Design review of the part built by this model. Coordinates are the model's own, in mm. A direction names the side the tool comes from. Round coordinates to 2 decimals unless told otherwise and drop trailing zeros. Loops run counter-clockwise (first coordinate to the right, second up) from the corner with the lowest first, then second, coordinate; pieces in that order, holes last. Notation, with made-up numbers: M 83.5,74 L 90.5,74 A25 ccw 90.5,95 Z; hole C -9.5,-4 d2. An arc over 180 degrees is marked long. One line per item, written item: value. Start each with the question number.
Item 1: We need section B-B (z = 26.5). Write out the cut boundary in (x, y), then the cut area to 3 significant figures.
Item 2: We need section A-A (x = -42.5). Write out the cut boundary in (y, z).
Item 3: Clearance check with flat-ended pins moving along their axes: pin 1 (12 mm diameter, centred on x = 9.5, z = 99.5, fed in from -Y); pin 2 (6 mm diameter, centred on y = -5.5, z = -70.5, fed in from +X); pin 3 (3 mm diameter, centred on x = 64.5, y = -5, fed in from +Z). State where each tip first meets the part, or that it passes through.
Item 4: For line 1 along Z through (x, y) = (101, -2.75); line 2 along Y through (x, z) = (-25, -11), list the stretches that pass through material, from the lowest coordinate up.
Item 5: For faces 1 (the flat face through (15, -8, 62)), 2 (the flat face through (-62, -8, -15)), 3 (the flat face through (-15, -8, 62)), 4 (the flat face through (63, -8, -15)), list the 3-axis set-ups (+Z, -Z, +X, -X, +Y, -Y) from which the entire face can be reached by the end or side of a thin tool; tool diameter is ignored.
from build123d import *

# Parameters (mm, degrees)
F0_W      = 30
F0_H      = 30
F1_DEPTH  = 20
F5_W      = 20
F5_H      = 30
F6_DEPTH  = 110
F4_W      = 30
F4_H      = 20
F7_DEPTH  = 110
F3_W      = 20
F3_H      = 30
F8_DEPTH  = 110
F2_W      = 30
F2_H      = 20
F9_DEPTH  = 110
F10_SIZE2 = 10
F10_SIZE  = 110
F11_R     = 14.99999


# Not quite as in the source:
# - a fillet or chamfer is up to 0.001 mm smaller than in the source, because OpenCascade refuses the exact size


with BuildPart() as f1:
    # F0 (on Front) → F1 (new body)
    with BuildSketch(Plane.XZ):
        Rectangle(F0_W, F0_H)
    extrude(amount=F1_DEPTH)

    # F5 (on face) → F6 (join)
    with BuildSketch(Plane.YZ.offset(15)):
        with Locations((-10, 0)):
            Rectangle(F5_W, F5_H)
    extrude(amount=F6_DEPTH)

    # F4 (on face) → F7 (join)
    with BuildSketch(Plane.XY.offset(15)):
        with Locations((0, -10)):
            Rectangle(F4_W, F4_H)
    extrude(amount=F7_DEPTH)

    # F3 (on face) → F8 (join)
    with BuildSketch(Plane(origin=(-15, 0, 0), x_dir=(0, -1, 0), z_dir=(-1, 0, 0))):
        with Locations((10, 0)):
            Rectangle(F3_W, F3_H)
    extrude(amount=F8_DEPTH)

    # F2 (on face) → F9 (join)
    with BuildSketch(Plane(origin=(0, 0, -15), x_dir=(1, 0, 0), z_dir=(0, 0, -1))):
        with Locations((0, 10)):
            Rectangle(F2_W, F2_H)
    extrude(amount=F9_DEPTH)

    # F10
    f10_edges = [f1.edges().sort_by_distance(p)[0] for p in [
        (-125, -20, 0),
        (0, -20, -125),
        (125, -20, 0),
        (0, -20, 125),
    ]]
    f10_side = f1.faces().sort_by_distance((0, -20, 0))[0]
    chamfer(f10_edges, length=F10_SIZE, length2=F10_SIZE2, reference=f10_side)

    # F11 (radius 15 in the source; OpenCascade refuses exactly that, so slightly less here)
    f11_edges = [f1.edges().sort_by_distance(p)[0] for p in [
        (15, -5, 125),
        (-15, -5, 125),
        (-125, -5, 15),
        (-125, -5, -15),
        (-15, -5, -125),
        (15, -5, -125),
        (125, -5, -15),
        (125, -5, 15),
    ]]
    fillet(f11_edges, radius=F11_R)


solid = f1.part
A:
1. outline: M -15,-18.95 L 15,-18.95 L 15,0 L -15,0 Z
1. area: 569 mm2
2. outline: M -17.5,-15 L 0,-15 L 0,15 L -17.5,15 Z
3. pin 1: y = -12.86
3. pin 2: x = 15
3. pin 3: z = 15
4. line 1: -15 to 15
4. line 2: -19.09 to 0
5. face 1: +Z, +X, +Y, -Y
5. face 2: -Z, -X, +Y, -Y
5. face 3: +Z, -X, +Y, -Y
5. face 4: -Z, +X, +Y, -Y
